Job drawing, mm, ordinate dimensions from the low corner. One solid piece. A direction names the side the tool comes from. Round coordinates to 2 decimals unless told otherwise and drop trailing zeros. Write each loop counter-clockwise with the first axis right and the second up, starting at its lowest first coordinate (ties: lowest second). Pieces come first, ordered by that corner, then holes. Notation, with made-up numbers: M 33.25,76.25 L 49.25,76.25 A15 ccw 49.25,88.25 Z; hole C 40,41 d3. An arc over 180 degrees is marked long. Answer as a JSON object with one key per item and string values. Group by question number.
1. Drill centre lines: line 1 (Z direction, x = 7, y = 4.25) (1 decimal); line 2 (Z direction, x = 10.75, y = 2.25) (1 decimal); line 3 (Z direction, x = 11.25, y = 0.5) (1 decimal). Where is each one in solid material? Low to high. Write a range as from..to.
2. Band-saw the part on A-A, the plane x = 11.25. Count the separate pieces of the cut face and the enclosed holes in it.
3. Two-plate mould, pull along Z, no slides. Class the marked faces 6 and 7: +Z half, -Z half, draft (parallel to the pull), parting line (faces both ways), or undercut.
4. Band-saw the part on B-B, the plane y = 3.5. Write the cut outline in (x, z) (1 decimal).
5. Which spindle directions (+Z, -Z, +X, -X, +Y, -Y) get a long thin tool onto all of the face, cutting with end or side? Do the marked faces 1, 2, 3, 4 and 5. Say none if no direction does.
6. Drop flat-ended pins along their axis: pin 1 (1.3 mm diameter, centred on x = 0.5, y = 2.5, fed in from -Z); pin 2 (1 mm diameter, centred on y = 1, z = 13.5, fed in from -X); pin 3 (3 mm diameter, centred on x = 10, z = 1.5, fed in from +Y). Give the stop position or say it passes through.
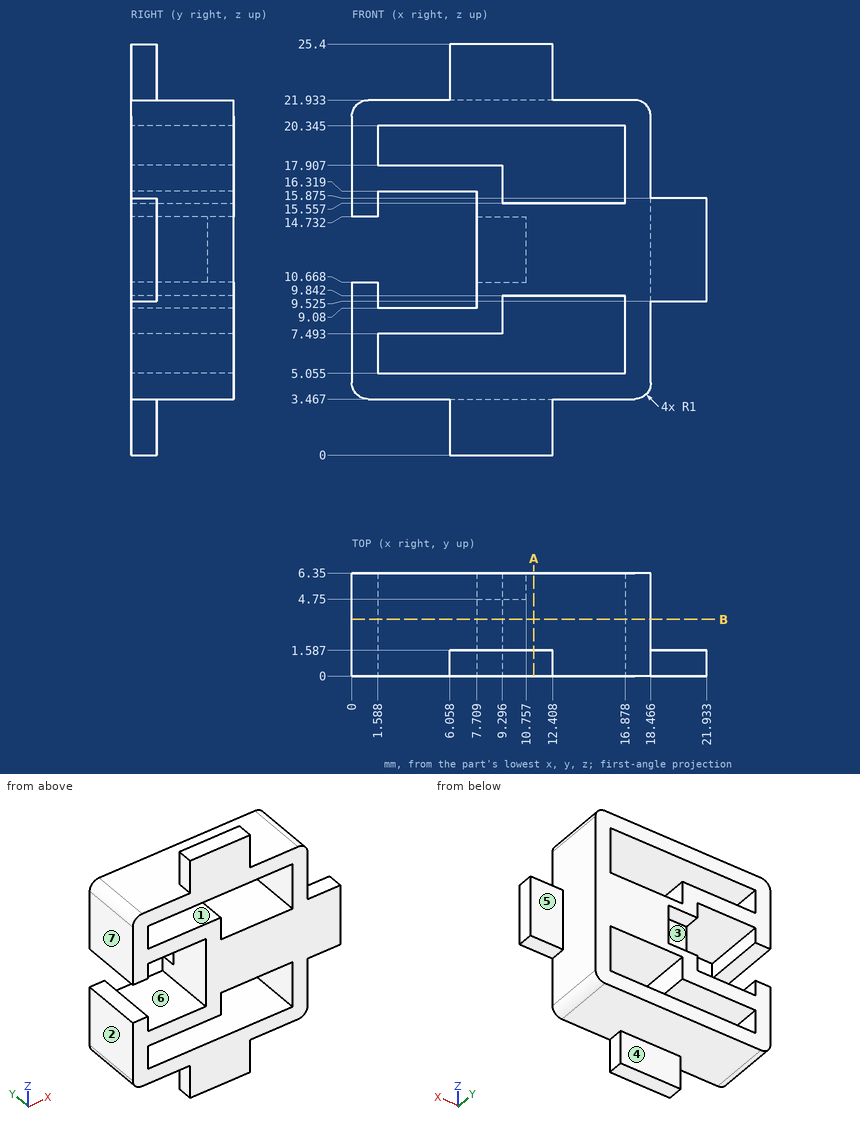
Worked answers:
{
 "1": {"line 1": "z = 3.5..5.1, 7.5..9.1, 16.3..17.9, 20.3..21.9", "line 2": "z = 3.5..5.1, 9.8..15.6, 20.3..21.9", "line 3": "z = 0..5.1, 9.8..15.6, 20.3..25.4"},
 "2": {"separate pieces": "3", "enclosed holes": "0"},
 "3": {"face 6": "undercut", "face 7": "draft"},
 "4": {"outline": "M 0,4.5 A1 ccw 1,3.5 L 17.5,3.5 A1 ccw 18.5,4.5 L 18.5,20.9 A1 ccw 17.5,21.9 L 1,21.9 A1 ccw 0,20.9 L 0,14.7 L 1.6,14.7 L 1.6,16.3 L 7.7,16.3 L 7.7,9.1 L 1.6,9.1 L 1.6,10.7 L 0,10.7 Z; hole M 1.6,5.1 L 16.9,5.1 L 16.9,9.8 L 9.3,9.8 L 9.3,7.5 L 1.6,7.5 Z; hole M 1.6,17.9 L 9.3,17.9 L 9.3,15.6 L 16.9,15.6 L 16.9,20.3 L 1.6,20.3 Z"},
 "5": {"face 1": "+Y, -Y", "face 2": "+Z, -Z, -X, +Y, -Y", "face 3": "-X, +Y", "face 4": "-Z, +X, -X, +Y", "face 5": "+Z, -Z, +X, +Y"},
 "6": {"pin 1": "stops at z = 3.47", "pin 2": "stops at x = 7.71", "pin 3": "stops at y = 1.59"}
}
